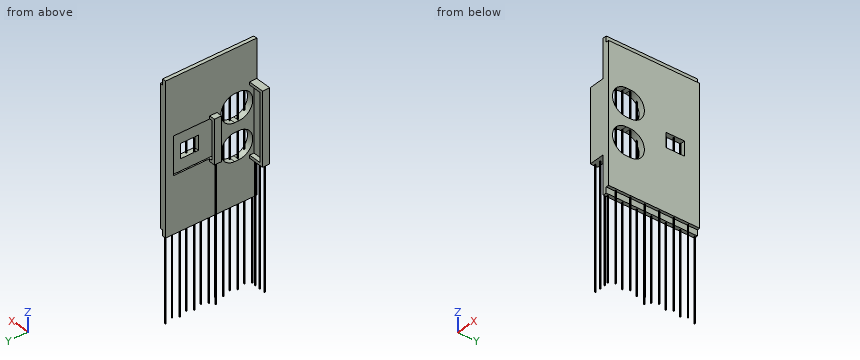
from build123d import *

# Parameters (mm, degrees)
SKETCH_1_W          = 2.5
SKETCH_1_H          = 103
SKETCH_1_W_2        = 2
SKETCH_1_H_2        = 95
EXTRUDE_1_DEPTH     = 63
SKETCH_5_W          = 50
SKETCH_5_H          = 2
EXTRUDE_2_DEPTH     = 11
EXTRUDE_3_DEPTH     = 3
CUT_EXTRUDE_1_DEPTH = 4.5
SKETCH_11_W         = 8.5
SKETCH_11_H         = 11.5
CUT_EXTRUDE_2_DEPTH = 4.5
SKETCH_12_W         = 26
SKETCH_12_H         = 28
SKETCH_12_W_2       = 25
SKETCH_12_H_2       = 27
SKETCH_12_W_3       = 8.5
SKETCH_12_H_3       = 11.5
CUT_EXTRUDE_3_DEPTH = 1
SKETCH_13_W         = 30
SKETCH_13_H         = 2
EXTRUDE_4_DEPTH     = 4
EXTRUDE_5_DEPTH     = 3
SKETCH_15_W         = 10
SKETCH_15_H         = 13
CUT_EXTRUDE_5_DEPTH = 10
EXTRUDE_START       = -73.34
SKETCH_16_W         = 0.5
SKETCH_16_H         = 0.5
EXTRUDE_6_DEPTH     = 130.501615
EXTRUDE_START_2     = -69.328472
SKETCH_17_W         = 0.5
SKETCH_17_H         = 0.5
EXTRUDE_7_DEPTH     = 130.490087
SKETCH_18_W         = 0.5
SKETCH_18_H         = 0.5
EXTRUDE_8_DEPTH     = 83.66161453
SKETCH_19_W         = 0.5
SKETCH_19_H         = 0.5
EXTRUDE_9_DEPTH     = 93.66161453


with BuildPart() as part:
    # 스케치1 → 보스-돌출1 (new body)
    with BuildSketch(Plane(origin=(0, 0, 0), x_dir=(1, 0, 0), z_dir=(0, 1, 0))):
        with Locations((-1, 0)):
            Rectangle(SKETCH_1_W, SKETCH_1_H)
        with Locations((1.25, 0)):
            Rectangle(SKETCH_1_W_2, SKETCH_1_H_2)
    extrude(amount=EXTRUDE_1_DEPTH)

    # 스케치5 → 보스-돌출2 (add)
    with BuildSketch(Plane.ZY.offset(2.25)):
        with Locations((0, 1)):
            Rectangle(SKETCH_5_W, SKETCH_5_H)
    extrude(amount=EXTRUDE_2_DEPTH)

    # 스케치7 → 보스-돌출3 (add)
    with BuildSketch(Plane(origin=(0, 2, 0), x_dir=(1, 0, 0), z_dir=(0, 1, 0))):
        Polygon((-2.25, 23), (-11.25, 23), (-11.25, -23), (-2.25, -23), (-2.25, -25), (-13.25, -25), (-13.25, 25), (-2.25, 25), align=None)
    extrude(amount=EXTRUDE_3_DEPTH)

    # 스케치10 → 컷-돌출1 (cut)
    with BuildSketch(Plane(origin=(2.25, 0, 0), x_dir=(0, 0, -1), z_dir=(1, 0, 0))):
        with BuildLine():
            Line((-21.84, 15.25), (-21.84, 12.25))
            ThreePointArc((-21.84, 12.25), (-12.34, 2.75), (-2.84, 12.25))
            Line((-2.84, 12.25), (-2.84, 15.25))
            ThreePointArc((-2.84, 15.25), (-12.34, 24.75), (-21.84, 15.25))
        make_face()
        with BuildLine():
            Line((3.66, 15.25), (3.66, 12.25))
            ThreePointArc((3.66, 12.25), (13.16, 2.75), (22.66, 12.25))
            Line((22.66, 12.25), (22.66, 15.25))
            ThreePointArc((22.66, 15.25), (13.16, 24.75), (3.66, 15.25))
        make_face()
    extrude(amount=-CUT_EXTRUDE_1_DEPTH, mode=Mode.SUBTRACT)

    # 스케치11 → 컷-돌출2 (cut)
    with BuildSketch(Plane.ZY.offset(2.25)):
        with Locations((0, 46.05)):
            Rectangle(SKETCH_11_W, SKETCH_11_H)
    extrude(amount=-CUT_EXTRUDE_2_DEPTH, mode=Mode.SUBTRACT)

    # 스케치12 → 컷-돌출3 (cut)
    # profile 1 of 2: a face of its own
    with BuildSketch(Plane.ZY.offset(2.25)):
        with Locations((0, 43.5)):
            Rectangle(SKETCH_12_W, SKETCH_12_H)
        with Locations((0, 43.5)):
            Rectangle(SKETCH_12_W_2, SKETCH_12_H_2, mode=Mode.SUBTRACT)
    # profile 2 of 2: a face of its own
    with BuildSketch(Plane.ZY.offset(2.25)):
        with Locations((0, 43.5)):
            Rectangle(SKETCH_12_W_2, SKETCH_12_H_2)
        with Locations((0, 46.05)):
            Rectangle(SKETCH_12_W_3, SKETCH_12_H_3, mode=Mode.SUBTRACT)
    extrude(amount=-CUT_EXTRUDE_3_DEPTH, mode=Mode.SUBTRACT)

    # 스케치13 → 보스-돌출4 (add)
    with BuildSketch(Plane.ZY.offset(2.25)):
        with Locations((0, 28.5)):
            Rectangle(SKETCH_13_W, SKETCH_13_H)
    extrude(amount=EXTRUDE_4_DEPTH)

    # 스케치14 → 보스-돌출5 (add)
    with BuildSketch(Plane(origin=(0, 29.5, 0), x_dir=(1, 0, 0), z_dir=(0, 1, 0))):
        Polygon((-2.25, -13), (-2.25, -15), (-6.25, -15), (-6.25, 15), (-2.25, 15), (-2.25, 13), (-4.25, 13), (-4.25, -13), align=None)
    extrude(amount=EXTRUDE_5_DEPTH)

    # 스케치15 → 컷-돌출5 (cut)
    with BuildSketch(Plane(origin=(2.25, 0, 0), x_dir=(0, 0, -1), z_dir=(1, 0, 0))):
        with Locations((0, 46.05)):
            Rectangle(SKETCH_15_W, SKETCH_15_H)
    extrude(amount=-CUT_EXTRUDE_5_DEPTH, mode=Mode.SUBTRACT)

    # 스케치16 → 보스-돌출6 (add)
    with BuildSketch(Plane(origin=(0, 0, -51.5), x_dir=(-1, 0, 0), z_dir=(0, 0, -1)).offset(EXTRUDE_START)):
        with Locations((1, 2.138286898)):
            Rectangle(SKETCH_16_W, SKETCH_16_H)
        with Locations((1, 12.138286898)):
            Rectangle(SKETCH_16_W, SKETCH_16_H)
        with Locations((1, 22.138286898)):
            Rectangle(SKETCH_16_W, SKETCH_16_H)
        with Locations((1, 32.138286898)):
            Rectangle(SKETCH_16_W, SKETCH_16_H)
        with Locations((1, 42.138286898)):
            Rectangle(SKETCH_16_W, SKETCH_16_H)
        with Locations((1, 52.138286898)):
            Rectangle(SKETCH_16_W, SKETCH_16_H)
        with Locations((1, 62.138286898)):
            Rectangle(SKETCH_16_W, SKETCH_16_H)
    extrude(amount=EXTRUDE_6_DEPTH)

    # 스케치17 → 보스-돌출7 (add)
    with BuildSketch(Plane(origin=(0, 0, -47.5), x_dir=(-1, 0, 0), z_dir=(0, 0, -1)).offset(EXTRUDE_START_2)):
        with Locations((-1, 5.967868798)):
            Rectangle(SKETCH_17_W, SKETCH_17_H)
        with Locations((-1, 15.967868798)):
            Rectangle(SKETCH_17_W, SKETCH_17_H)
        with Locations((-1, 25.967868798)):
            Rectangle(SKETCH_17_W, SKETCH_17_H)
        with Locations((-1, 35.967868798)):
            Rectangle(SKETCH_17_W, SKETCH_17_H)
        with Locations((-1, 45.967868798)):
            Rectangle(SKETCH_17_W, SKETCH_17_H)
        with Locations((-1, 55.967868798)):
            Rectangle(SKETCH_17_W, SKETCH_17_H)
    extrude(amount=EXTRUDE_7_DEPTH)

    # 스케치18 → 보스-돌출8 (add)
    with BuildSketch(Plane(origin=(0, 0, -25), x_dir=(-1, 0, 0), z_dir=(0, 0, -1))):
        with Locations((3.97675174, 2.5)):
            Rectangle(SKETCH_18_W, SKETCH_18_H)
        with Locations((7.97675174, 2.5)):
            Rectangle(SKETCH_18_W, SKETCH_18_H)
        with Locations((11.97675174, 2.5)):
            Rectangle(SKETCH_18_W, SKETCH_18_H)
    extrude(amount=EXTRUDE_8_DEPTH)

    # 스케치19 → 보스-돌출9 (add)
    with BuildSketch(Plane(origin=(0, 0, -15), x_dir=(-1, 0, 0), z_dir=(0, 0, -1))):
        with Locations((4.25, 30)):
            Rectangle(SKETCH_19_W, SKETCH_19_H)
    extrude(amount=EXTRUDE_9_DEPTH)


solid = part.part
Model file for the job. Use its own axes, mm. Give positions to 0.01 mm unless a question says otherwise; leave off trailing zeros. Order: outer loops, then holes, each group sorted by start corner. A loop starts at its lowest first (then second) coordinate and runs counter-clockwise, first axis right, second up. Notation, with made-up numbers: M -27.5,79 L -3.5,79 A29 ccw -3.5,102 Z; hole C -33,43.5 d8. An arc over 180 degrees is marked long. Put each result on its own line as item: value. Start each with the question number.
(1) Band-saw the part on B-B on z = -68. Count the separate pieces of the cut face and the enclosed holes in it, then the cut area to 3 significant figures.
(2) Band-saw the part on A-A on z = -38. Give the cut face in (x, y), then the cut area to 4 significant figures.
(3) Drill centre lines: L1, parallel to Z at x = 0.5, y = 41; L2, parallel to Z at x = 0.5, y = 33; L3, parallel to X at y = 18, z = 24. Where is each one in solid material? Low to high. Write a range as [from, to].
(4) Pin check, flat tips, straight feed: pin 1 Ø2.5 at (x, y) = (0, 14) entering from -Z; pin 2 Ø4 at (y, z) = (35, -68) entering from -X; pin 3 Ø2 at (x, z) = (0, -62) entering from +Y; pin 4 Ø2 at (y, z) = (14.5, 6.5) entering from -X. Stop position of each tip, or through.
Results below:
1. separate pieces: 17
1. enclosed holes: 0
1. area: 4.25 mm2
2. outline: M -12.23,2.25 L -11.73,2.25 L -11.73,2.75 L -12.23,2.75 Z; M -8.23,2.25 L -7.73,2.25 L -7.73,2.75 L -8.23,2.75 Z; M -4.5,29.75 L -4,29.75 L -4,30.25 L -4.5,30.25 Z; M -4.23,2.25 L -3.73,2.25 L -3.73,2.75 L -4.23,2.75 Z; M -2.25,0 L 2.25,0 L 2.25,63 L -2.25,63 Z
2. area: 284.5 mm2
3. L1: z = [-47.5, -5], [5, 47.5]
3. L2: z = [-47.5, 47.5]
3. L3: x = [-2.25, 2.25]
4. pin 1: stops at z = -51.5
4. pin 2: stops at x = 0.75
4. pin 3: stops at y = 62.39
4. pin 4: passes through
